Part model, mm, in its own coordinate system. A direction names the side the tool comes from. Round coordinates to 2 decimals unless told otherwise and drop trailing zeros. Loops run counter-clockwise (first coordinate to the right, second up) from the corner with the lowest first, then second, coordinate; pieces in that order, holes last.
(1) Cut at B-B on y = 5. List the corners of the cut face in (x, z), then the cut area to 3 significant figures.
(2) Cut at A-A on x = 5. List the corners of the cut face in (y, z).
(3) Mould opens along X. For faces 1 (the face through (11.8, 33, 3.8)), 2 (the face through (15.8, -5, -0.6)), 3 (the face through (0, 3, 0)), 4 (the face through (4, -3, 4)) say: +X half, -X half, draft (parallel to the pull), parting line (faces both ways), or undercut.
(4) Tool access for faces 5 (the face through (6.8, -5, -0.6)), 6 (the face through (13, -3, 4)), 7 (the face through (-11, 10.5, 5)), 8 (the face through (11, 9.75, -6)): list every direction of +Z, -Z, +X, -X, +Y, -Y with a clear straight run to the whole face (end or side of a thin tool).
(5) Cut at C-C on z = -3. Count the separate pieces of the cut face and the enclosed holes in it, then the cut area to 3 significant figures.
(6) Flat gauge pins, fed straight in: pin 1 (2 mm diameter, centred on x = -11, y = 12.5, fed in from +Z) (3 decimals); pin 2 (6 mm diameter, centred on y = -9, z = -2, fed in from +X); pin 3 (4 mm diameter, centred on x = -11, y = 34.5, fed in from -Z); pin 4 (1.5 mm diameter, centred on x = -18, z = 2.5, fed in from -Y). Where does each tip first touch, or does it go through?
(7) Probe probe 1 along Y at (x, z) = (-11, 3.8); probe 2 along X at (y, z) = (-5, 0.25); probe 3 along Z at (x, y) = (-15, 23). List the from-to ranges inside material, lowest first.
from build123d import *

# Parameters (mm, degrees)
SKETCH1_W            = 46.2
SKETCH1_H            = 16
BOSS_EXTRUDE1_DEPTH  = 43
SKETCH2_W            = 4.6
SKETCH2_H            = 12
BOSS_EXTRUDE2_DEPTH  = 7
SKETCH8_R            = 6
BOSS_EXTRUDE3_DEPTH  = 4.6
LPATTERN1_COUNT      = 4
LPATTERN1_PITCH      = 9
SKETCH4_R            = 2.1
CUT_EXTRUDE1_DEPTH   = 39.9
SKETCH6_W            = 40.6
SKETCH6_H            = 4.4
CUT_EXTRUDE2_DEPTH   = 40
SKETCH9_R            = 1.7
CUT_EXTRUDE3_DEPTH   = 17
FILLET2_R            = 2
CUT_EXTRUDE4_DEPTH   = 4
LPATTERN2_COUNT      = 2
LPATTERN2_PITCH      = 22
LPATTERN2_COUNT_DIR2 = 2
LPATTERN2_PITCH_DIR2 = 22
SKETCH11_R           = 3
CUT_EXTRUDE5_DEPTH   = 3


with BuildPart() as part:
    # Sketch1 → Boss-Extrude1 (new body)
    with BuildSketch(Plane(origin=(0, 0, 0), x_dir=(1, 0, 0), z_dir=(0, 1, 0))):
        Rectangle(SKETCH1_W, SKETCH1_H)
    extrude(amount=BOSS_EXTRUDE1_DEPTH)

    # Sketch2 → Boss-Extrude2 (add)
    with BuildSketch(Plane.XZ):
        with Locations((13.5, -2)):
            Rectangle(SKETCH2_W, SKETCH2_H)
    boss_extrude2 = extrude(amount=BOSS_EXTRUDE2_DEPTH)

    # Sketch8 → Boss-Extrude3 (add)
    with BuildSketch(Plane(origin=(15.8, 0, 0), x_dir=(0, 0, -1), z_dir=(1, 0, 0))):
        with Locations((2, -7)):
            Circle(SKETCH8_R)
    boss_extrude3 = extrude(amount=-BOSS_EXTRUDE3_DEPTH)

    # LPattern1: Boss-Extrude2, Boss-Extrude3 ×4
    with Locations(*[(-i * LPATTERN1_PITCH, 0, 0) for i in range(1, LPATTERN1_COUNT)]):
        add(boss_extrude2)
        add(boss_extrude3)

    # Sketch4 → Cut-Extrude1 (cut, through all)
    with BuildSketch(Plane(origin=(15.8, 0, 0), x_dir=(0, 0, -1), z_dir=(1, 0, 0))):
        with Locations((2, -7)):
            Circle(SKETCH4_R)
    extrude(amount=-CUT_EXTRUDE1_DEPTH, mode=Mode.SUBTRACT)

    # Sketch6 → Cut-Extrude2 (cut)
    with BuildSketch(Plane(origin=(0, 43, 0), x_dir=(1, 0, 0), z_dir=(0, 1, 0))):
        with Locations((0, -0.4)):
            Rectangle(SKETCH6_W, SKETCH6_H)
    extrude(amount=-CUT_EXTRUDE2_DEPTH, mode=Mode.SUBTRACT)

    # Sketch9 → Cut-Extrude3 (cut, through all)
    with BuildSketch(Plane.XY.offset(8)):
        with Locations((11, 12.5)):
            Circle(SKETCH9_R)
        with Locations((-11, 12.5)):
            Circle(SKETCH9_R)
        with Locations((11, 34.5)):
            Circle(SKETCH9_R)
        with Locations((-11, 34.5)):
            Circle(SKETCH9_R)
    extrude(amount=-CUT_EXTRUDE3_DEPTH, mode=Mode.SUBTRACT)

    # Fillet2
    fillet2_edges = [part.edges().sort_by_distance(p)[0] for p in [
        (-23.1, 21.5, -8),
        (23.1, 21.5, -8),
        (23.1, 21.5, 8),
        (-23.1, 21.5, 8),
    ]]
    fillet(fillet2_edges, radius=FILLET2_R)

    # Sketch10 → Cut-Extrude4 (cut)
    with BuildSketch(Plane(origin=(0, 0, -8), x_dir=(-1, 0, 0), z_dir=(0, 0, -1))):
        Polygon((12.58771324, 9.75), (9.41228676, 9.75), (7.824573519, 12.5), (9.41228676, 15.25), (12.58771324, 15.25), (14.175426481, 12.5), align=None)
    cut_extrude4 = extrude(amount=-CUT_EXTRUDE4_DEPTH, mode=Mode.SUBTRACT)

    # LPattern2: Cut-Extrude4 2 × 2
    with Locations(*[(j * LPATTERN2_PITCH_DIR2, i * LPATTERN2_PITCH, 0) for i in range(LPATTERN2_COUNT) for j in range(LPATTERN2_COUNT_DIR2) if (i, j) != (0, 0)]):
        add(cut_extrude4, mode=Mode.SUBTRACT)

    # Sketch11 → Cut-Extrude5 (cut)
    with BuildSketch(Plane.XY.offset(8)):
        with Locations((11, 12.5)):
            Circle(SKETCH11_R)
        with Locations((-11, 12.5)):
            Circle(SKETCH11_R)
        with Locations((-11, 34.5)):
            Circle(SKETCH11_R)
        with Locations((11, 34.5)):
            Circle(SKETCH11_R)
    extrude(amount=-CUT_EXTRUDE5_DEPTH, mode=Mode.SUBTRACT)


solid = part.part
Final values:
1. outline: (-23.1, -6) arc R2 ccw to (-21.1, -8) - (21.1, -8) arc R2 ccw to (23.1, -6) - (23.1, 6) arc R2 ccw to (21.1, 8) - (-21.1, 8) arc R2 ccw to (-23.1, 6) - close; hole (-20.3, -1.8) - (20.3, -1.8) - (20.3, 2.6) - (-20.3, 2.6) - close
1. area: 557 mm2
2. outline: (-7, -8) - (43, -8) - (43, -1.8) - (3, -1.8) - (3, 2.6) - (43, 2.6) - (43, 8) - (0, 8) - (0, 4) - (-7, 4) arc R6 ccw to start; hole circle Ø4.2 at (-7, -2)
3. face 1: undercut
3. face 2: +X half
3. face 3: undercut
3. face 4: draft
4. face 5: +Z, -Z, -Y
4. face 6: +Z, +X, -X, -Y
4. face 7: +Z
4. face 8: -Z
5. separate pieces: 5
5. enclosed holes: 4
5. area: 2,120 mm2
6. pin 1: passes through
6. pin 2: stops at x = 15.8
6. pin 3: stops at z = -4
6. pin 4: stops at y = 0
7. probe 1: y = 0 to 10.8, 14.2 to 32.8, 36.2 to 43
7. probe 2: x = -15.8 to -11.2, -6.8 to -2.2, 2.2 to 6.8, 11.2 to 15.8
7. probe 3: z = -8 to -1.8, 2.6 to 8
